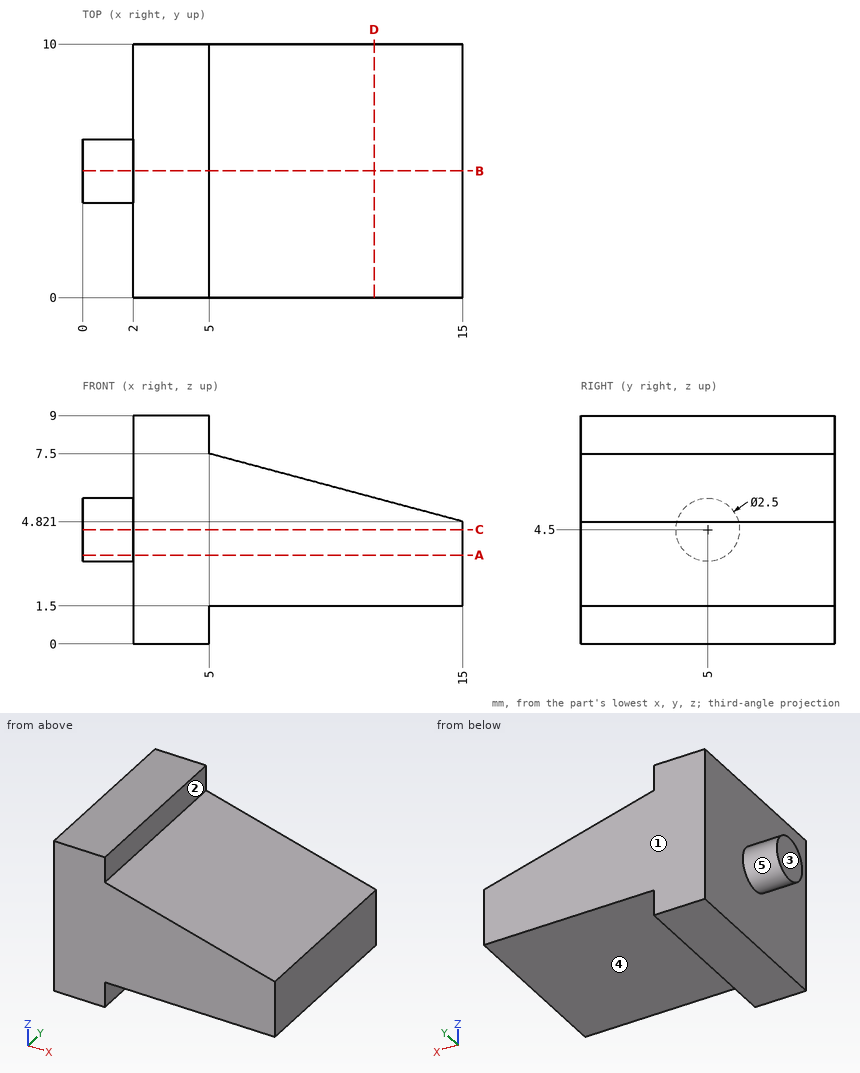
Input: dimensioned drawing with shaded views. Units: mm. Origin: part minimum x, y, z. A direction names the side the tool comes from. Round coordinates to 2 decimals unless told otherwise and drop trailing zeros. Write each loop counter-clockwise with the first axis right and the second up, starting at its lowest first coordinate (ties: lowest second). Pieces come first, ordered by that corner, then holes. Notation, with made-up numbers: (36.5, 56) - (90.5, 56) arc R16 ccw to (90.5, 75) - close; hole circle Ø3 at (-26.75, 12). An arc over 180 degrees is marked (long way). Write item = value, one per line.
(1) Section query C-C on z = 4.5. Output: boundary loops of the cut face in (x, y).
Geometry check:
outline = (0, 3.75) - (2, 3.75) - (2, 0) - (15, 0) - (15, 10) - (2, 10) - (2, 6.25) - (0, 6.25) - close
(2) Section query B-B on y = 5. Output: boundary loops of the cut face in (x, z).
Geometry check:
outline = (0, 3.25) - (2, 3.25) - (2, 0) - (5, 0) - (5, 1.5) - (15, 1.5) - (15, 4.82) - (5, 7.5) - (5, 9) - (2, 9) - (2, 5.75) - (0, 5.75) - close
(3) Material intervals for probe 1 along X at (y, z) = (1.5, 4.75); probe 2 along X at (y, z) = (6.75, 1); probe 3 along Z at (x, y) = (7.5, 6.5), sorted ascending.
Geometry check:
probe_1 = 2 to 15
probe_2 = 2 to 5
probe_3 = 1.5 to 6.83
(4) Access query for the marked faces 1, 2, 3, 4 and 5. Directions: +Z, -Z, +X, -X, +Y, -Y. A direction counts if a zero-diameter tool reaches every point of the face in a straight line with its end or side. Return the directions, or none.
Geometry check:
face_1 = +Z, -Z, +X, -X, +Y
face_2 = +Z, +X, +Y, -Y
face_3 = +Z, -Z, -X, +Y, -Y
face_4 = -Z, +X, +Y, -Y
face_5 = -X
(5) Section query D-D on x = 11.5. Output: boundary loops of the cut face in (y, z).
Geometry check:
outline = (0, 1.5) - (10, 1.5) - (10, 5.76) - (0, 5.76) - close
(6) Contact query for flat-ended pins moving along their axis: pin 1 Ø3 at (x, y) = (8.5, 3) entering from -Z; pin 2 Ø4 at (y, z) = (2.5, 2) entering from -X. Output: stop coordinate, or through.
Geometry check:
pin_1 = 1.5
pin_2 = 2
(7) Section query A-A on z = 3.5. Output: boundary loops of the cut face in (x, y).
Geometry check:
outline = (0, 4.25) - (2, 4.25) - (2, 0) - (15, 0) - (15, 10) - (2, 10) - (2, 5.75) - (0, 5.75) - close
